Part model, mm, in its own coordinate system. A direction names the side the tool comes from. Coordinates: 2 decimals unless noted, no trailing zeros. Loops run counter-clockwise (first coordinate to the right, second up) from the corner with the lowest first, then second, coordinate; pieces in that order, holes last. Notation, with made-up numbers: (50, -28) -> (80, -28) arc R27 cw to (80, -2) -> close; hole circle Ø1 at (45, 62). An arc over 180 degrees is marked (long way). Use one line per item in the form item = value. Start each with the question number.
(1) Band-saw the part on A-A on x = 0. Give the cut face in (y, z), then the cut area to 3 significant figures.
(2) Band-saw the part on D-D on x = -18. Give the cut face in (y, z), then the cut area to 3 significant figures.
(3) Band-saw the part on C-C on z = -1.75. Give the cut face in (x, y), then the cut area to 3 significant figures.
(4) Drill centre lines: L1, parallel to Y at x = 0, z = -1.5; L2, parallel to Y at x = 0, z = -0.75; L3, parallel to Y at x = 0, z = 1.3. Where is each one in solid material? Low to high. Write a range as [from, to].
(5) 3-axis set-ups, long thin cutter, end or side, ignore diameter. For faces 1 (the cylindrical face through (3, 0, -2)), 2 (the cylindrical face through (-16.845, -0.479, -1.479)): which of +Z, -Z, +X, -X, +Y, -Y reach the whole face in a straight line?
(6) Pin check, flat tips, straight feed: P1, Ø4, axis at x = 0, y = 18, coming from the +Z side; P2, Ø5, axis at x = 0, y = 0, coming from the +Z side; P3, Ø1, axis at x = 1.5, z = 1.5, coming from the +Y side; P4, Ø2, axis at x = 0, y = -18, coming from the +Z side. Stop position of each tip, or through.
(7) Mould opens along Y. For faces 3 (the cylindrical face through (-0.59, -4.46, 1.38)), 4 (the cylindrical face through (0.672, -16.946, -1.479)), 5 (the flat face through (0, -2, 2.8)), 6 (the cylindrical face through (-0.27, 16.78, -1.48)) say: +Y half, -Y half, draft (parallel to the pull), parting line (faces both ways), or undercut.
Autodesk Inventor part; units mm, degrees
ref_plane "YZ Plane" through (0, 0, 0) normal (1, 0, 0) x (0, 1, 0)
ref_plane "XZ Plane" through (0, 0, 0) normal (0, 1, 0) x (-1, 0, 0)
ref_plane "XY Plane" through (0, 0, 0) normal (0, 0, 1) x (1, 0, 0)
sketch "스케치1" plane through (0, 0, 0) normal (0, 0, 1) x (1, 0, 0)
  circle A0 centre (0, 0) radius 24.5
  circle A1 centre (0, 0) radius 4.5
  circle A2 centre (0, 0) radius 1.75
  circle A3 centre (0, 18) radius 1.25
  circle A4 centre (-18, 0) radius 1.25
  circle A5 centre (0, -18) radius 1.25
  circle A6 centre (18, 0) radius 1.25
  dimension "d0" = 49
  dimension "d1" = 9
  dimension "d2" = 3.5
  dimension "d7" = 2.5
  dimension "d8" = 18
  dimension "d11" = 360
extrude "돌출1" add sketch "스케치1" against normal blind 3 contours A0 | A1
extrude "돌출2" add sketch "스케치1" along normal blind 2.8 contours A1
sketch "스케치2" plane through (0, 0, -3) normal (0, 0, -1) x (-1, 0, 0)
  circle A0 centre (0, 0) radius 3
  dimension "d13" = 6
extrude "돌출3" cut sketch "스케치2" against normal blind 2
properties part number "좌측 축"
A:
q1.outline = (-24.5, -3) -> (-19.25, -3) -> (-19.25, 0) -> (-24.5, 0) -> close; (-16.75, -3) -> (-3, -3) -> (-3, -1) -> (-1.75, -1) -> (-1.75, 2.8) -> (-4.5, 2.8) -> (-4.5, 0) -> (-16.75, 0) -> close; (1.75, -1) -> (3, -1) -> (3, -3) -> (16.75, -3) -> (16.75, 0) -> (4.5, 0) -> (4.5, 2.8) -> (1.75, 2.8) -> close; (19.25, -3) -> (24.5, -3) -> (24.5, 0) -> (19.25, 0) -> close
q1.area = 132 mm²
q2.outline = (-16.62, -3) -> (-1.25, -3) -> (-1.25, 0) -> (-16.62, 0) -> close; (1.25, -3) -> (16.62, -3) -> (16.62, 0) -> (1.25, 0) -> close
q2.area = 92.2 mm²
q3.outline = circle Ø49 at (0, 0); hole circle Ø2.5 at (-18, 0); hole circle Ø6 at (0, 0); hole circle Ø2.5 at (0, -18); hole circle Ø2.5 at (0, 18); hole circle Ø2.5 at (18, 0)
q3.area = 1,840 mm²
q4.L1 = [-24.5, -19.25], [-16.75, -3], [3, 16.75], [19.25, 24.5]
q4.L2 = [-24.5, -19.25], [-16.75, -1.75], [1.75, 16.75], [19.25, 24.5]
q4.L3 = [-4.5, -1.75], [1.75, 4.5]
q5.face_1 = -Z
q5.face_2 = +Z, -Z
q6.P1 = 0
q6.P2 = 2.8
q6.P3 = 4.39
q6.P4 = through
q7.face_3 = parting line
q7.face_4 = undercut
q7.face_5 = draft
q7.face_6 = undercut
